The model under review builds one solid part; all positions refer to its coordinate system, in mm. A direction names the side the tool comes from. Coordinates: 2 decimals unless noted, no trailing zeros. Order: outer loops, then holes, each group sorted by start corner. A loop starts at its lowest first (then second) coordinate and runs counter-clockwise, first axis right, second up. Notation, with made-up numbers: (13, 14) -> (29, 14) arc R16 cw to (29, 32) -> close; hole circle Ø4 at (3, 70.5). An arc over 180 degrees is marked (long way). Put each result on its own line as item: value.
from build123d import *
from OCP.BRepFilletAPI import BRepFilletAPI_MakeChamfer

# Parameters (mm, degrees)
BOSS_EXTRUDE1_DEPTH   = 5
CHAMFER1_SIZE         = 5
CHAMFER1_SIZE2        = 5.047084744
FILLET4_R             = 20
F_4_0MM_DOWEL_HOLE1_D = 4
SKETCH5_R             = 2.75
CUT_EXTRUDE1_DEPTH    = 2
FILLET5_R             = 30
FILLET6_R             = 20
FILLET7_R             = 40
FILLET8_R             = 20
FILLET9_R             = 5
CUT_EXTRUDE3_REACH    = 154.398
SKETCH7_R             = 1.5
CUT_EXTRUDE4_REACH    = 154.398
SKETCH8_W             = 23.5
SKETCH8_H             = 12.4
CUT_EXTRUDE5_REACH    = 154.398
SKETCH9_R             = 1.1
CUT_EXTRUDE6_REACH    = 154.398
SKETCH11_R            = 1.6


with BuildPart() as part:
    # Sketch1 → Boss-Extrude1 (new body)
    with BuildSketch(Plane(origin=(0, 0, 0), x_dir=(1, 0, 0), z_dir=(0, 1, 0))):
        Polygon((40, 60), (70, 60), (90, 25), (90, -25), (70, -60), (40, -60), (10, -35), (-10, -35), (-40, -60), (-120, -60), (-140, -50), (-140, 50), (-120, 60), (-40, 60), (-10, 35), (10, 35), align=None)
    extrude(amount=BOSS_EXTRUDE1_DEPTH)

    # Chamfer1: one chamfer whose edges measure the first distance from different faces: ONE call of the kernel's chamfer builder (chamfer() names one face for all edges)
    chamfer1_edges_1 = [part.edges().sort_by_distance(p)[0] for p in [
        (-40, 2.5, 60),
    ]]
    chamfer1_side_1 = [part.faces().sort_by_distance(p)[0] for p in [
        (-80, 2.5, 60),
    ]]
    chamfer1_edges_2 = [part.edges().sort_by_distance(p)[0] for p in [
        (-40, 2.5, -60),
    ]]
    chamfer1_side_2 = [part.faces().sort_by_distance(p)[0] for p in [
        (-25, 2.5, -47.5),
    ]]
    chamfer1 = BRepFilletAPI_MakeChamfer(part.part.solid().wrapped)
    for e in chamfer1_edges_1:
        chamfer1.Add(CHAMFER1_SIZE, CHAMFER1_SIZE2, e.wrapped, chamfer1_side_1[0].wrapped)  # the first distance lies on this face
    for e in chamfer1_edges_2:
        chamfer1.Add(CHAMFER1_SIZE, CHAMFER1_SIZE2, e.wrapped, chamfer1_side_2[0].wrapped)  # the first distance lies on this face
    add(Compound.cast(chamfer1.Shape()), mode=Mode.REPLACE)

    # Fillet4
    fillet4_edges = [part.edges().sort_by_distance(p)[0] for p in [
        (40, 2.5, -60),
        (70, 2.5, -60),
        (70, 2.5, 60),
        (40, 2.5, 60),
    ]]
    fillet(fillet4_edges, radius=FILLET4_R)

    # Ø4.0mm Dowel Hole1 (through all)
    with Locations(Plane(origin=(52.817273997, 5, -52), x_dir=(0, 0, 1), z_dir=(0, 1, 0))):
        with Locations((0, 0), (104, 0)):
            Hole(F_4_0MM_DOWEL_HOLE1_D / 2)

    # Sketch5 → Cut-Extrude1 (cut)
    with BuildSketch(Plane.XZ):
        with Locations(Location((52.817273997, 52, 0), (0, 0, 270))):
            Circle(SKETCH5_R)
        with Locations(Location((52.817273997, -52, 0), (0, 0, 270))):
            Circle(SKETCH5_R)
    extrude(amount=-CUT_EXTRUDE1_DEPTH, mode=Mode.SUBTRACT)

    # Fillet5
    fillet5_edges = [part.edges().sort_by_distance(p)[0] for p in [
        (90, 2.5, -25),
        (90, 2.5, 25),
    ]]
    fillet(fillet5_edges, radius=FILLET5_R)

    # Fillet6
    fillet6_edges = [part.edges().sort_by_distance(p)[0] for p in [
        (10, 2.5, 35),
        (10, 2.5, -35),
    ]]
    fillet(fillet6_edges, radius=FILLET6_R)

    # Fillet7
    # the kernel refuses this fillet: 40 mm, written as the material it adds along each edge
    with BuildSketch(Plane(origin=(-10, 0, -35), x_dir=(-0.768221279597376, 0, -0.6401843996644798), z_dir=(0, 1, 0))) as fillet7_piece_1:
        with BuildLine():
            CenterArc((14.420794682, -40), FILLET7_R, 90, 37.26938559)
            Line((-9.801736302, -8.168113585), (0, 0))
            Line((0, 0), (14.420794682, 0))
        make_face()
    extrude(amount=5)
    with BuildSketch(Plane(origin=(-10, 0, 35), x_dir=(1, 0, 0), z_dir=(0, 1, 0))) as fillet7_piece_2:
        with BuildLine():
            CenterArc((14.529014643, -39.96081897), FILLET7_R, 92.536185502, 37.26938559)
            Line((-11.078361343, -9.231967786), (0, 0))
            Line((0, 0), (12.759001296, 0))
        make_face()
    extrude(amount=5)

    # Fillet8
    fillet8_edges = [part.edges().sort_by_distance(p)[0] for p in [
        (-120, 2.5, 60),
        (-120, 2.5, -60),
    ]]
    fillet(fillet8_edges, radius=FILLET8_R)

    # Fillet9
    fillet9_edges = [part.edges().sort_by_distance(p)[0] for p in [
        (-140, 2.5, 50),
        (-140, 2.5, -50),
    ]]
    fillet(fillet9_edges, radius=FILLET9_R)

    # Sketch7 → Cut-Extrude3 (cut, up to next)
    with BuildSketch(Plane(origin=(0, 5, 0), x_dir=(1, 0, 0), z_dir=(0, 1, 0)), mode=Mode.PRIVATE) as cut_extrude3_sk1:
        with Locations(Location((-110.27864045, 40, 0), (0, 0, 270))):
            Circle(SKETCH7_R)
    cut_extrude3_tool1 = extrude(cut_extrude3_sk1.sketch, amount=-CUT_EXTRUDE3_REACH, mode=Mode.PRIVATE) & part.part
    # Sketch7 → Cut-Extrude3 (cut, up to next)
    with BuildSketch(Plane(origin=(0, 5, 0), x_dir=(1, 0, 0), z_dir=(0, 1, 0)), mode=Mode.PRIVATE) as cut_extrude3_sk2:
        with Locations(Location((-80.57864045, 40, 0), (0, 0, 270))):
            Circle(SKETCH7_R)
    cut_extrude3_tool2 = extrude(cut_extrude3_sk2.sketch, amount=-CUT_EXTRUDE3_REACH, mode=Mode.PRIVATE) & part.part
    cut_extrude3_1 = cut_extrude3_tool1.solids().sort_by_distance((-110.27864, 5, -40))[0]
    add(cut_extrude3_1, mode=Mode.SUBTRACT)
    cut_extrude3_2 = cut_extrude3_tool2.solids().sort_by_distance((-80.57864, 5, -40))[0]
    add(cut_extrude3_2, mode=Mode.SUBTRACT)
    cut_extrude3 = cut_extrude3_1 + cut_extrude3_2  # Cut-Extrude3 as one shape, for the pattern or mirror that repeats it

    # Mirror1: Cut-Extrude3 across plane
    add(cut_extrude3.mirror(Plane.XY), mode=Mode.SUBTRACT)

    # Sketch8 → Cut-Extrude4 (cut, up to next)
    with BuildSketch(Plane(origin=(0, 5, 0), x_dir=(1, 0, 0), z_dir=(0, 1, 0)), mode=Mode.PRIVATE) as cut_extrude4_sk1:
        with Locations((57.85, 0)):
            Rectangle(SKETCH8_W, SKETCH8_H)
    cut_extrude4_tool1 = extrude(cut_extrude4_sk1.sketch, amount=-CUT_EXTRUDE4_REACH, mode=Mode.PRIVATE) & part.part
    add(cut_extrude4_tool1.solids().sort_by_distance((57.85, 5, 0))[0], mode=Mode.SUBTRACT)

    # Sketch9 → Cut-Extrude5 (cut, up to next)
    with BuildSketch(Plane(origin=(0, 5, 0), x_dir=(1, 0, 0), z_dir=(0, 1, 0)), mode=Mode.PRIVATE) as cut_extrude5_sk1:
        with Locations(Location((-90.57864045, 25, 0), (0, 0, 270))):
            Circle(SKETCH9_R)
    cut_extrude5_tool1 = extrude(cut_extrude5_sk1.sketch, amount=-CUT_EXTRUDE5_REACH, mode=Mode.PRIVATE) & part.part
    # Sketch9 → Cut-Extrude5 (cut, up to next)
    with BuildSketch(Plane(origin=(0, 5, 0), x_dir=(1, 0, 0), z_dir=(0, 1, 0)), mode=Mode.PRIVATE) as cut_extrude5_sk2:
        with Locations(Location((-56.57864045, 25, 0), (0, 0, 270))):
            Circle(SKETCH9_R)
    cut_extrude5_tool2 = extrude(cut_extrude5_sk2.sketch, amount=-CUT_EXTRUDE5_REACH, mode=Mode.PRIVATE) & part.part
    # Sketch9 → Cut-Extrude5 (cut, up to next)
    with BuildSketch(Plane(origin=(0, 5, 0), x_dir=(1, 0, 0), z_dir=(0, 1, 0)), mode=Mode.PRIVATE) as cut_extrude5_sk3:
        with Locations(Location((-90.57864045, -25, 0), (0, 0, 270))):
            Circle(SKETCH9_R)
    cut_extrude5_tool3 = extrude(cut_extrude5_sk3.sketch, amount=-CUT_EXTRUDE5_REACH, mode=Mode.PRIVATE) & part.part
    # Sketch9 → Cut-Extrude5 (cut, up to next)
    with BuildSketch(Plane(origin=(0, 5, 0), x_dir=(1, 0, 0), z_dir=(0, 1, 0)), mode=Mode.PRIVATE) as cut_extrude5_sk4:
        with Locations(Location((-56.57864045, -25, 0), (0, 0, 270))):
            Circle(SKETCH9_R)
    cut_extrude5_tool4 = extrude(cut_extrude5_sk4.sketch, amount=-CUT_EXTRUDE5_REACH, mode=Mode.PRIVATE) & part.part
    add(cut_extrude5_tool1.solids().sort_by_distance((-90.57864, 5, -25))[0], mode=Mode.SUBTRACT)
    add(cut_extrude5_tool2.solids().sort_by_distance((-56.57864, 5, -25))[0], mode=Mode.SUBTRACT)
    add(cut_extrude5_tool3.solids().sort_by_distance((-90.57864, 5, 25))[0], mode=Mode.SUBTRACT)
    add(cut_extrude5_tool4.solids().sort_by_distance((-56.57864, 5, 25))[0], mode=Mode.SUBTRACT)

    # Sketch11 → Cut-Extrude6 (cut, up to next)
    with BuildSketch(Plane(origin=(0, 5, 0), x_dir=(1, 0, 0), z_dir=(0, 1, 0)), mode=Mode.PRIVATE) as cut_extrude6_sk1:
        with Locations(Location((82, 24, 0), (0, 0, 270))):
            Circle(SKETCH11_R)
    cut_extrude6_tool1 = extrude(cut_extrude6_sk1.sketch, amount=-CUT_EXTRUDE6_REACH, mode=Mode.PRIVATE) & part.part
    # Sketch11 → Cut-Extrude6 (cut, up to next)
    with BuildSketch(Plane(origin=(0, 5, 0), x_dir=(1, 0, 0), z_dir=(0, 1, 0)), mode=Mode.PRIVATE) as cut_extrude6_sk2:
        with Locations(Location((82, -24, 0), (0, 0, 270))):
            Circle(SKETCH11_R)
    cut_extrude6_tool2 = extrude(cut_extrude6_sk2.sketch, amount=-CUT_EXTRUDE6_REACH, mode=Mode.PRIVATE) & part.part
    add(cut_extrude6_tool1.solids().sort_by_distance((82, 5, -24))[0], mode=Mode.SUBTRACT)
    add(cut_extrude6_tool2.solids().sort_by_distance((82, 5, 24))[0], mode=Mode.SUBTRACT)


solid = part.part
Item 1: For line 1 (Z direction, x = 49, y = 3.9); line 2 (Z direction, x = 82, y = 2.9); line 3 (Z direction, x = -90, y = 3.15), list the stretches that pass through material, from the lowest coordinate up. Write a range as from..to.
Answers below:
line 1: -60..-6.2, 6.2..60
line 2: -39..-25.6, -22.4..22.4, 25.6..39
line 3: -60..-25.94, -24.06..24.06, 25.94..60
Item 2: Consider section D-D on x = -12.5. Write out the cut boundary in (y, z).
Answers below:
outline: (0, -38.77) -> (5, -38.77) -> (5, 38.77) -> (0, 38.77) -> close
Item 3: For faces 4 (the cylindrical face through (9.66, 2.54, 36.23)), 5 (the flat face through (-40.665, 2.465, -58.422)), 6 (the cylindrical face through (52.938, 0.986, -49.253)), 7 (the flat face through (58, 3, -6.2)), list the 3-axis set-ups (+Z, -Z, +X, -X, +Y, -Y) from which the entire face can be reached by the end or side of a thin tool; tool diameter is ignored.
Answers below:
face 4: +Z, +Y, -Y
face 5: -Z, +Y, -Y
face 6: -Y
face 7: +Y, -Y
Item 4: For pin 1 Ø2 at (x, y) = (27.5, 2) entering from +Z; pin 2 Ø2.5 at (x, z) = (-80.58, -40) entering from -Y; pin 3 Ø4.5 at (x, z) = (52.82, 52) entering from -Y; pin 4 Ø3 at (x, y) = (24, 4) entering from -Z, all flat-tipped, find the tip position at first contact; note any pin that passes through.
Answers below:
pin 1: z = 50.42
pin 2: through
pin 3: y = 2
pin 4: z = -47.92
Item 5: Mouldability with a two-part tool opening along X and no side actions: class faces 1 (the flat face through (69.6, 3, 0)), 2 (the cylindrical face through (-119.81, 2.54, 59.48)), 3 (the cylindrical face through (68.304, 2.535, 57.372)) as +X half, -X half, draft (parallel to the pull), parting line (faces both ways), or undercut.
Answers below:
face 1: undercut
face 2: -X half
face 3: +X half
Item 6: Consider section B-B on y = 2.95. Count the separate pieces of the cut face and the enclosed holes in it, and give its area (3 significant figures).
Answers below:
separate pieces: 1
enclosed holes: 13
area: 23,800 mm^2
Item 7: Consider section A-A on x = 64. Write out the cut boundary in (y, z), and give its area (3 significant figures).
Answers below:
outline: (0, -59.2) -> (5, -59.2) -> (5, -6.2) -> (0, -6.2) -> close; (0, 6.2) -> (5, 6.2) -> (5, 59.2) -> (0, 59.2) -> close
area: 530 mm^2
Item 8: Consider section C-C on x = -41.5. Write out the cut boundary in (y, z), and give its area (3 significant figures).
Answers below:
outline: (0, -58.72) -> (5, -58.72) -> (5, 58.73) -> (0, 58.73) -> close
area: 587 mm^2
